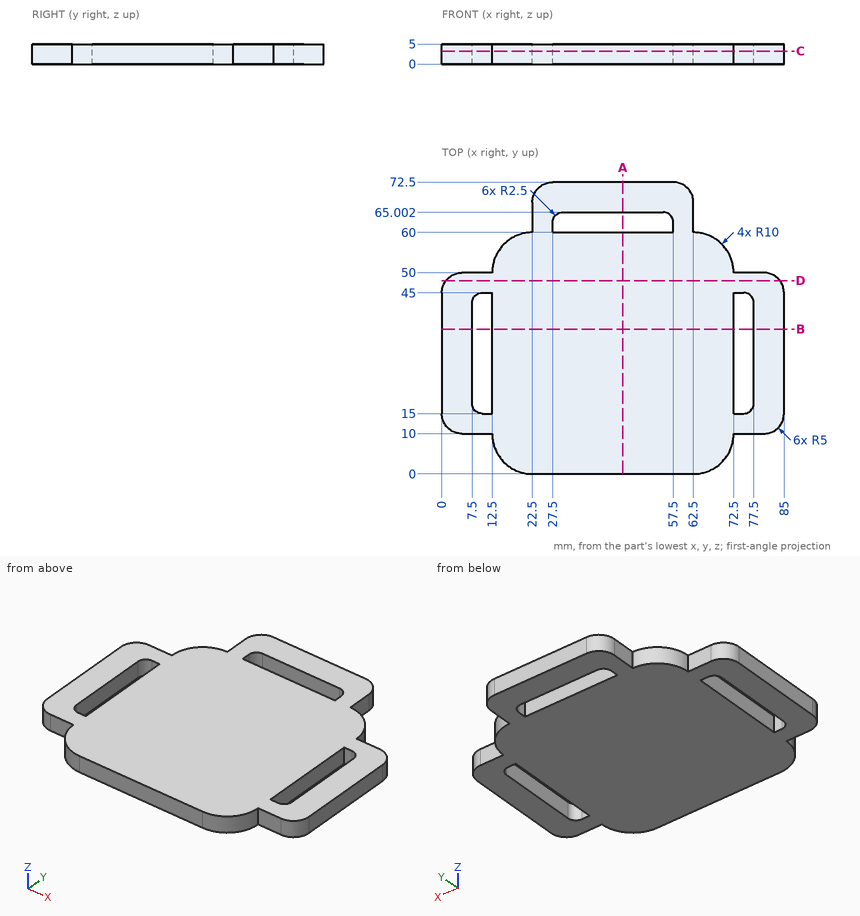
Drawing for the job (mm, zero at the part's lowest x, y, z). Give positions to 0.01 mm unless a question says otherwise; leave off trailing zeros. Order: outer loops, then holes, each group sorted by start corner. A loop starts at its lowest first (then second) coordinate and runs counter-clockwise, first axis right, second up. Notation, with made-up numbers: (59.5, 50.25) - (107.5, 50.25) arc R7 ccw to (107.5, 57.25) - close; hole circle Ø4 at (17, 48.5). An arc over 180 degrees is marked (long way). Use one line per item in the form item = value.
Item 1: Slice it at B-B on y = 36. Give the cut face in (x, z).
Solution:
outline = (0, 0) - (7.5, 0) - (7.5, 5) - (0, 5) - close; (12.5, 0) - (72.5, 0) - (72.5, 5) - (12.5, 5) - close; (77.5, 0) - (85, 0) - (85, 5) - (77.5, 5) - close
Item 2: Slice it at C-C on z = 3.2. Count the separate pieces of the cut face and the enclosed holes in it, and give its area (3 significant figures).
Solution:
separate_pieces = 1
enclosed_holes = 3
area = 4,540 mm2
Item 3: Slice it at A-A on x = 45. Give the cut face in (y, z).
Solution:
outline = (0, 0) - (60, 0) - (60, 5) - (0, 5) - close; (65, 0) - (72.5, 0) - (72.5, 5) - (65, 5) - close
Item 4: Probe probe 1 along X at (y, z) = (34, 3.8); probe 2 along Y at (x, z) = (52, 1.4); probe 3 along Y at (x, z) = (11.5, 1.85). List the from-to ranges inside material, lowest first. Write a range as from..to.
Solution:
probe_1 = 0..7.5, 12.5..72.5, 77.5..85
probe_2 = 0..60, 65..72.5
probe_3 = 10..15, 45..50
Item 5: Slice it at D-D on y = 48. Give the cut face in (x, z).
Solution:
outline = (1, 0) - (84, 0) - (84, 5) - (1, 5) - close
Item 6: Pin check, flat tips, straight feed: pin 1 Ø0.8 at (y, z) = (60.5, 3) entering from -X; pin 2 Ø2 at (y, z) = (52.5, 3.5) entering from -X; pin 3 Ø0.8 at (y, z) = (61, 1.5) entering from +X; pin 4 Ø2.5 at (y, z) = (23.5, 2.5) entering from -X. Stop position of each tip, or through.
Solution:
pin_1 = 22.5
pin_2 = 12.61
pin_3 = 62.5
pin_4 = 0
